CAD build for the part. Positions are in the model's coordinates, mm. Face numbers are marked on the shaded views. A direction names the side the tool comes from. Round coordinates to 2 decimals unless told otherwise and drop trailing zeros. Order: outer loops, then holes, each group sorted by start corner. A loop starts at its lowest first (then second) coordinate and runs counter-clockwise, first axis right, second up. Notation, with made-up numbers: M 83.5,75 L 133.5,75 A26 cw 133.5,111 Z; hole C -15,-5.75 d1. An arc over 180 degrees is marked long. Answer as a JSON object with one key per item and string values.
```python
from build123d import *

# Parameters (mm, degrees)
SKETCH1_W          = 50.8
SKETCH1_H          = 12.7
BASE_EXTRUDE_DEPTH = 6.35
FILLET1_R          = 6.35
SHELL1_DEPTH       = 6.35
SHELL1_START       = -1.905
SHELL1_2_DEPTH     = 10.16
SHELL1_3_DEPTH     = 1.905
SHELL1_START_2     = 6.35
SHELL1_4_DEPTH     = 1.905
FILLET3_R          = 3.175
FILLET4_R          = 1.778


# Read off the part's stored shape, not the designer's step: Shell1
# Some blends are built 0.0001 mm under size
with BuildPart() as part:
    # Sketch1 → Base-Extrude (new body)
    with BuildSketch(Plane.XY):
        with Locations((25.4, 6.35)):
            Rectangle(SKETCH1_W, SKETCH1_H)
    extrude(amount=BASE_EXTRUDE_DEPTH)

    # Fillet1
    fillet1_edges = [part.edges().sort_by_distance(p)[0] for p in [
        (0, 0, 3.175),
        (0, 12.7, 3.175),
    ]]
    fillet(fillet1_edges, radius=FILLET1_R - 0.0001)  # a hair under: the kernel refuses the full size

    # Shell1 outline → Shell1 (cut)
    with BuildSketch(Plane.XY):
        with BuildLine():
            Line((6.35, 0), (50.8, 0))
            Line((50.8, 0), (50.8, 12.7))
            Line((50.8, 12.7), (6.35, 12.7))
            ThreePointArc((6.35, 12.7), (1.859871939, 10.840128061), (0, 6.35))
            ThreePointArc((0, 6.35), (1.859871939, 1.859871939), (6.35, 0))
        make_face()
    extrude(amount=SHELL1_DEPTH, mode=Mode.SUBTRACT)

    # Shell1 2 outline → Shell1 2 (add)
    with BuildSketch(Plane.XY.offset(SHELL1_START)):
        with BuildLine():
            Line((6.35, -1.905), (50.8, -1.905))
            Line((50.8, -1.905), (50.8, 0))
            Line((50.8, 0), (6.35, 0))
            ThreePointArc((6.35, 0), (1.859871939, 1.859871939), (0, 6.35))
            ThreePointArc((0, 6.35), (1.859871939, 10.840128061), (6.35, 12.7))
            Line((6.35, 12.7), (50.8, 12.7))
            Line((50.8, 12.7), (50.8, 14.605))
            Line((50.8, 14.605), (6.35, 14.605))
            ThreePointArc((6.35, 14.605), (0.512833521, 12.187166479), (-1.905, 6.35))
            ThreePointArc((-1.905, 6.35), (0.512833521, 0.512833521), (6.35, -1.905))
        make_face()
    extrude(amount=SHELL1_2_DEPTH)

    # Shell1 3 outline → Shell1 3 (add)
    with BuildSketch(Plane.XY.offset(SHELL1_START)):
        with BuildLine():
            Line((6.35, 0), (50.8, 0))
            Line((50.8, 0), (50.8, 12.7))
            Line((50.8, 12.7), (6.35, 12.7))
            ThreePointArc((6.35, 12.7), (1.859871939, 10.840128061), (0, 6.35))
            ThreePointArc((0, 6.35), (1.859871939, 1.859871939), (6.35, 0))
        make_face()
    extrude(amount=SHELL1_3_DEPTH)

    # Shell1 4 outline → Shell1 4 (add)
    with BuildSketch(Plane.XY.offset(SHELL1_START_2)):
        with BuildLine():
            Line((6.35, 0), (50.8, 0))
            Line((50.8, 0), (50.8, 12.7))
            Line((50.8, 12.7), (6.35, 12.7))
            ThreePointArc((6.35, 12.7), (1.859871939, 10.840128061), (0, 6.35))
            ThreePointArc((0, 6.35), (1.859871939, 1.859871939), (6.35, 0))
        make_face()
    extrude(amount=SHELL1_4_DEPTH)

    # Fillet3
    fillet3_edges = [part.edges().sort_by_distance(p)[0] for p in [
        (28.575, -1.905, -1.905),
        (0.512833521, 0.512833521, -1.905),
        (0.512833521, 12.187166479, -1.905),
        (28.575, -1.905, 8.255),
        (0.512833521, 0.512833521, 8.255),
        (0.512833521, 12.187166479, 8.255),
        (28.575, 14.605, -1.905),
        (28.575, 14.605, 8.255),
    ]]
    fillet(fillet3_edges, radius=FILLET3_R)

    # Fillet4
    # the kernel refuses this fillet: 1.778 mm, written as the material it takes off along each edge
    with BuildSketch(Plane(origin=(50.8, -1.905, 1.27), x_dir=(0, 1, 0), z_dir=(0, 0, 1))) as fillet4_piece_1:
        with BuildLine():
            CenterArc((FILLET4_R, FILLET4_R), FILLET4_R, 180, 90)
            Line((0, FILLET4_R), (0, 0))
            Line((0, 0), (FILLET4_R, 0))
        make_face()
    extrude(amount=3.81, mode=Mode.SUBTRACT)
    with BuildSketch(Plane(origin=(50.8, 1.27, -1.905), x_dir=(0, 0, 1), z_dir=(0, 1, 0)), Plane(origin=(50.8, 11.43, 8.255), x_dir=(0, 0, -1), z_dir=(0, -1, 0))) as fillet4_piece_2:
        with BuildLine():
            CenterArc((FILLET4_R, -FILLET4_R), FILLET4_R, 90, 90)
            Line((0, -FILLET4_R), (0, 0))
            Line((0, 0), (FILLET4_R, 0))
        make_face()
    extrude(amount=10.16, mode=Mode.SUBTRACT)
    with BuildSketch(Plane(origin=(50.8, 14.605, 1.27), x_dir=(0, -1, 0), z_dir=(0, 0, 1))) as fillet4_piece_3:
        with BuildLine():
            CenterArc((FILLET4_R, -FILLET4_R), FILLET4_R, 90, 90)
            Line((0, -FILLET4_R), (0, 0))
            Line((0, 0), (FILLET4_R, 0))
        make_face()
    extrude(amount=3.81, mode=Mode.SUBTRACT)
    with BuildSketch(Plane(origin=(50.8, 11.43, 5.08), x_dir=(0, 1, 0), z_dir=(0, 0, -1))) as fillet4_piece_4:
        with BuildLine():
            CenterArc((3.175 - FILLET4_R, -FILLET4_R), FILLET4_R, 0, 90)
            Line((3.175, -FILLET4_R), (3.175, 0))
            Line((3.175, 0), (3.175 - FILLET4_R, 0))
        make_face()
    revolve(axis=Axis((50.8, 11.43, 5.08), (1, 0, 0)), revolution_arc=90, mode=Mode.SUBTRACT)
    with BuildSketch(Plane(origin=(50.8, 11.43, 1.27), x_dir=(0, 1, 0), z_dir=(0, 0, 1))) as fillet4_piece_5:
        with BuildLine():
            CenterArc((3.175 - FILLET4_R, FILLET4_R), FILLET4_R, 270, 90)
            Line((3.175, FILLET4_R), (3.175, 0))
            Line((3.175, 0), (3.175 - FILLET4_R, 0))
        make_face()
    revolve(axis=Axis((50.8, 11.43, 1.27), (-1, 0, 0)), revolution_arc=90, mode=Mode.SUBTRACT)
    with BuildSketch(Plane(origin=(50.8, 1.27, 5.08), x_dir=(0, -1, 0), z_dir=(0, 0, -1))) as fillet4_piece_6:
        with BuildLine():
            CenterArc((3.175 - FILLET4_R, FILLET4_R), FILLET4_R, 270, 90)
            Line((3.175, FILLET4_R), (3.175, 0))
            Line((3.175, 0), (3.175 - FILLET4_R, 0))
        make_face()
    revolve(axis=Axis((50.8, 1.27, 5.08), (-1, 0, 0)), revolution_arc=90, mode=Mode.SUBTRACT)
    with BuildSketch(Plane(origin=(50.8, 1.27, 1.27), x_dir=(0, -1, 0), z_dir=(0, 0, 1))) as fillet4_piece_7:
        with BuildLine():
            CenterArc((3.175 - FILLET4_R, -FILLET4_R), FILLET4_R, 0, 90)
            Line((3.175, -FILLET4_R), (3.175, 0))
            Line((3.175, 0), (3.175 - FILLET4_R, 0))
        make_face()
    revolve(axis=Axis((50.8, 1.27, 1.27), (1, 0, 0)), revolution_arc=90, mode=Mode.SUBTRACT)


solid = part.part
```
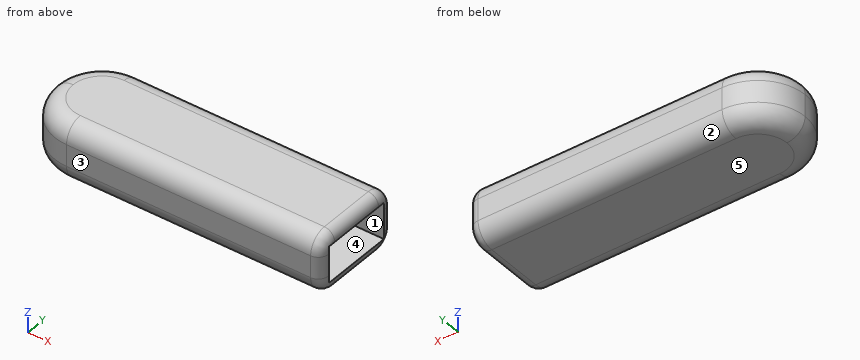
Item 1: Drop flat-ended pins along their axis: pin 1 Ø5 at (x, z) = (4, 6.5) entering from -Y; pin 2 Ø5 at (y, z) = (11, 4.5) entering from -X. Give the stop position or say it passes through.
Worked answers:
{"pin 1": "stops at y = -1.9", "pin 2": "stops at x = -1.62"}
Item 2: Saw through at B-B on z = 1.75. List the corners of the cut face in (x, y) (3 decimals), and give its area (3 significant figures).
Worked answers:
{"outline": "M 6.35,-1.905 L 49.022,-1.905 A1.778 ccw 50.8,-0.127 L 50.8,0 L 6.35,0 A6.35 cw 6.35,12.7 L 50.8,12.7 L 50.8,12.827 A1.778 ccw 49.022,14.605 L 6.35,14.605 A8.255 ccw Z", "area": "212 mm2"}
Item 3: Wall check: line 1 along Z through (x, y) = (4.5, 5.25) (3 decimals); line 2 along Y through (x, z) = (38, 3.5) (3 decimals); line 3 along Y through (x, z) = (3.5, 3.5). Give the ranges that are in metal, low to high. Write a range as [from, to].
Worked answers:
{"line 1": "z = [-1.905, 0], [6.35, 8.255]", "line 2": "y = [-1.905, 0], [12.7, 14.605]", "line 3": "y = [-1.4, 0.68], [12.02, 14.1]"}
Item 4: Two-plate mould, pull along Z, no slides. Class the marked faces 3, 4 and 5: released by +Z, released by -Z, zero draft, split by the parting line, or undercut.
Worked answers:
{"face 3": "zero draft", "face 4": "undercut", "face 5": "released by -Z"}
Item 5: Saw through at A-A on x = 32. List the corners of the cut face in (y, z) (3 decimals).
Worked answers:
{"outline": "M -1.905,1.27 A3.175 ccw 1.27,-1.905 L 11.43,-1.905 A3.175 ccw 14.605,1.27 L 14.605,5.08 A3.175 ccw 11.43,8.255 L 1.27,8.255 A3.175 ccw -1.905,5.08 Z; hole M 0,0 L 12.7,0 L 12.7,6.35 L 0,6.35 Z"}
Item 6: 3-axis set-ups, long thin cutter, end or side, ignore diameter. For the marked faces 1 and 2: which of +Z, -Z, +X, -X, +Y, -Y reach the whole face in a straight line?
Worked answers:
{"face 1": "+X", "face 2": "-Z, +X, -X, +Y"}
